Model file for the job. Use its own axes, mm. Face numbers are marked on the shaded views. Round coordinates to 2 decimals unless told otherwise and drop trailing zeros. Order: outer loops, then holes, each group sorted by start corner. A loop starts at its lowest first (then second) coordinate and runs counter-clockwise, first axis right, second up. Notation, with made-up numbers: (-3.5, 24.5) - (49.5, 24.5) arc R22 ccw to (49.5, 46.5) - close; hole circle Ø7 at (7, 11.25). An arc over 180 degrees is marked (long way). Put each result on its own line as item: value. Start each with the question number.
Item 1: Saw through at C-C on z = 2.5. List the corners of the cut face in (x, y).
Item 2: Saw through at A-A on y = 3. List the corners of the cut face in (x, z), plus the area to 3 significant figures.
Item 3: Pin check, flat tips, straight feed: pin 1 Ø0.8 at (x, y) = (-14, 10.5) entering from +Z; pin 2 Ø1.1 at (y, z) = (10.5, 6) entering from +X; pin 3 Ø4 at (x, y) = (-15.5, 7.5) entering from -Z. Stop position of each tip, or through.
Item 4: Saw through at D-D on z = -33.5. List the corners of the cut face in (x, y), plus the area to 3 significant figures.
Item 5: Mould opens along Z. For the marked faces 1 and 2 say: pulls with the +Z half, pulls with the -Z half, needs draft (parallel to the pull), parting line crosses it, or undercut.
Item 6: Saw through at B-B on x = 6. List the corners of the cut face in (y, z), plus the area to 3 significant figures.
Item 7: Probe probe 1 along Z at (x, y) = (-5, 3); probe 2 along X at (y, z) = (8.25, 9.5). List the from-to ranges inside material, lowest first.
```python
from build123d import *

# Parameters (mm, degrees)
SKETCH_4_W          = 51.2
SKETCH_4_H          = 51.2
CUT_EXTRUDE_1_DEPTH = 58.445626622
SKETCH_5_W          = 58.2
SKETCH_5_H          = 58.2
SKETCH_5_W_2        = 57.2
SKETCH_5_H_2        = 57.2
EXTRUDE_1_DEPTH     = 1


with BuildPart() as part:
    # Эскиз1 → По сечениям1 section 0
    with BuildSketch(Plane(origin=(0, 0, 0), x_dir=(1, 0, 0), z_dir=(0, 1, 0))):
        with BuildLine():
            Line((-40, -40), (40, -40))
            Line((40, -40), (40, 40))
            Line((40, 40), (-40, 40))
            Line((-40, 40), (-40, -40))
        make_face()
    # Эскиз2 → По сечениям1 section 1
    with BuildSketch(Plane(origin=(0, 5, 0), x_dir=(1, 0, 0), z_dir=(0, 1, 0))):
        with BuildLine():
            Line((-40, -40), (40, -40))
            Line((40, -40), (40, 40))
            Line((40, 40), (-40, 40))
            Line((-40, 40), (-40, -40))
        make_face()
    loft()

    # Эскиз2<3> → По сечениям2 section 0
    with BuildSketch(Plane(origin=(0, 5, 0), x_dir=(1, 0, 0), z_dir=(0, 1, 0))):
        with BuildLine():
            Line((-35, -35), (35, -35))
            Line((35, -35), (35, 35))
            Line((35, 35), (-35, 35))
            Line((-35, 35), (-35, -35))
        make_face()
    # Эскиз3 → По сечениям2 section 1
    with BuildSketch(Plane(origin=(0, 10, 0), x_dir=(1, 0, 0), z_dir=(0, 1, 0))):
        with BuildLine():
            Line((-35, -35), (35, -35))
            Line((35, -35), (35, 35))
            Line((35, 35), (-35, 35))
            Line((-35, 35), (-35, -35))
        make_face()
    loft()

    # Эскиз4 → Вырез-Вытянуть1 (cut, through all)
    with BuildSketch(Plane(origin=(0, 10, 0), x_dir=(1, 0, 0), z_dir=(0, 1, 0))):
        Rectangle(SKETCH_4_W, SKETCH_4_H)
    extrude(amount=-CUT_EXTRUDE_1_DEPTH, mode=Mode.SUBTRACT)

    # Эскиз5 → Бобышка-Вытянуть1 (add)
    with BuildSketch(Plane(origin=(0, 10, 0), x_dir=(1, 0, 0), z_dir=(0, 1, 0))):
        Rectangle(SKETCH_5_W, SKETCH_5_H)
        Rectangle(SKETCH_5_W_2, SKETCH_5_H_2, mode=Mode.SUBTRACT)
    extrude(amount=EXTRUDE_1_DEPTH)


solid = part.part
```
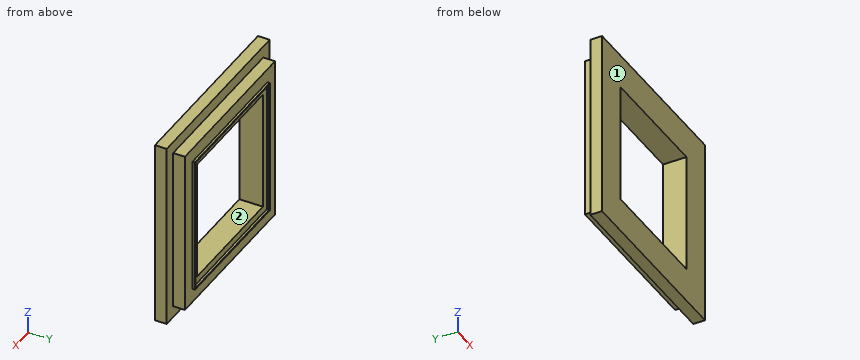
Results found:
1. outline: (-40, 0) - (-25.6, 0) - (-25.6, 10) - (-28.6, 10) - (-28.6, 11) - (-29.1, 11) - (-29.1, 10) - (-35, 10) - (-35, 5) - (-40, 5) - close; (25.6, 0) - (40, 0) - (40, 5) - (35, 5) - (35, 10) - (29.1, 10) - (29.1, 11) - (28.6, 11) - (28.6, 10) - (25.6, 10) - close
2. outline: (-40, -40) - (40, -40) - (40, 40) - (-40, 40) - close; hole (-25.6, -25.6) - (25.6, -25.6) - (25.6, 25.6) - (-25.6, 25.6) - close
2. area: 3,780 mm²
3. pin 1: stops at z = 29.1
3. pin 2: stops at x = 35
3. pin 3: stops at z = -35
4. outline: (-40, 0) - (40, 0) - (40, 5) - (35, 5) - (35, 10) - (-35, 10) - (-35, 5) - (-40, 5) - close
4. area: 750 mm²
5. face 1: needs draft
5. face 2: undercut
6. outline: (0, -40) - (5, -40) - (5, -35) - (10, -35) - (10, -29.1) - (11, -29.1) - (11, -28.6) - (10, -28.6) - (10, -25.6) - (0, -25.6) - close; (0, 25.6) - (10, 25.6) - (10, 28.6) - (11, 28.6) - (11, 29.1) - (10, 29.1) - (10, 35) - (5, 35) - (5, 40) - (0, 40) - close
6. area: 239 mm²
7. probe 1: z = -40 to -25.6, 25.6 to 40
7. probe 2: x = -35 to -25.6, 25.6 to 35
